For this review, use the dimensioned drawing (mm, ordinates from the lowest corner) and the shaded views. Coordinates: 2 decimals unless noted, no trailing zeros. Loops run counter-clockwise (first coordinate to the right, second up) from the corner with the lowest first, then second, coordinate; pieces in that order, holes last.
1. To check wall thickness, follow probe 1 along Z at (x, y) = (67, 10); probe 2 along Y at (x, z) = (91, 10.25); probe 3 along Z at (x, y) = (103.5, 5). State the ranges of each line that lie inside material, in increasing order.
2. Take a section at A-A, the plane y = 10. State the section outline as (x, z) points, then the cut area to 4 significant figures.
3. Clearance check with flat-ended pins moving along their axes: P1, Ø1, axis at x = 93, y = 8.5, coming from the -Z side; P2, Ø8, axis at y = 7.5, z = 11, coming from the -X side; P3, Ø5, axis at x = 59, y = 3.5, coming from the +Z side. State where each tip first meets the part, or that it passes through.
4. Take a section at C-C, the plane x = 31. State the section outline as (y, z) points.
5. Take a section at B-B, the plane z = 10. State the section outline as (x, y) points.
6. Take a section at D-D, the plane z = 17. State the section outline as (x, y) points, then the cut area to 3 significant figures.
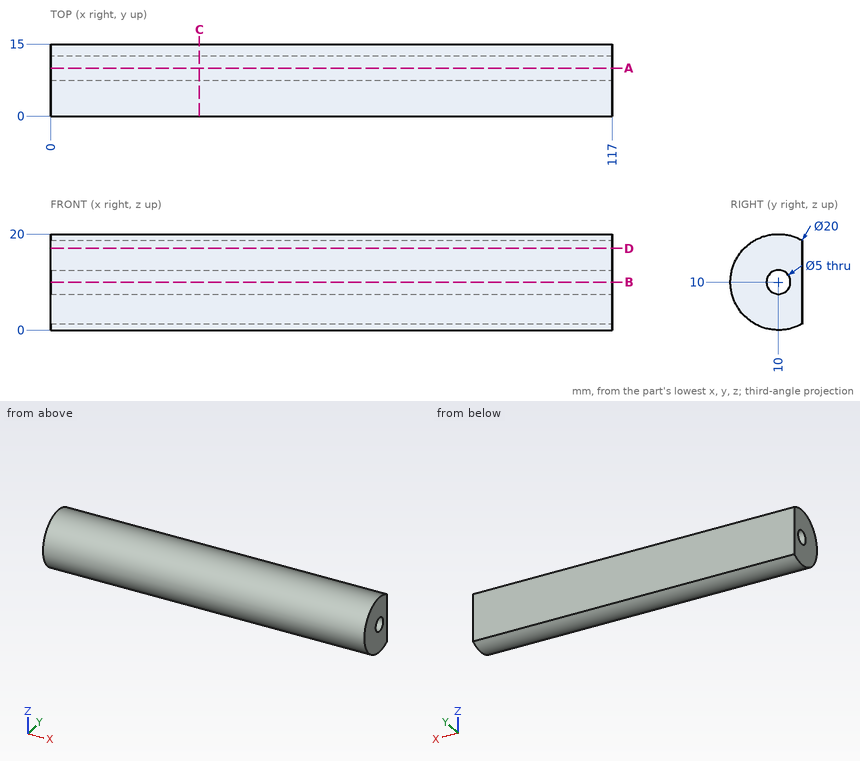
Results list:
1. probe 1: z = 0 to 7.5, 12.5 to 20
1. probe 2: y = 0 to 7.51, 12.49 to 15
1. probe 3: z = 1.34 to 18.66
2. outline: (0, 0) - (117, 0) - (117, 7.5) - (0, 7.5) - close; (0, 12.5) - (117, 12.5) - (117, 20) - (0, 20) - close
2. area: 1,755 mm2
3. P1: stops at z = 0.05
3. P2: stops at x = 0
3. P3: stops at z = 19.17
4. outline: (15, 1.34) - (15, 18.66) arc R10 ccw (long way) to start; hole circle Ø5 at (10, 10)
5. outline: (0, 0) - (117, 0) - (117, 7.5) - (0, 7.5) - close; (0, 12.5) - (117, 12.5) - (117, 15) - (0, 15) - close
6. outline: (0, 2.86) - (117, 2.86) - (117, 15) - (0, 15) - close
6. area: 1,420 mm2
